Part model, mm, in its own coordinate system. A direction names the side the tool comes from. Coordinates: 2 decimals unless noted, no trailing zeros. Order: outer loops, then holes, each group sorted by start corner. A loop starts at its lowest first (then second) coordinate and runs counter-clockwise, first axis right, second up. Notation, with made-up numbers: (-5, 53) - (3, 53) arc R23 cw to (3, 77) - close; hole circle Ø11 at (-13.75, -22.5). An arc over 180 degrees is marked (long way). Use a Markdown table: item, result. Add a question column.
1) Saw through at B-B on z = -1. List the corners of the cut face in (x, y) (1 decimal).
2) Wall check: L1, parallel to X at y = 35.5, z = -5.5; L2, parallel to X at y = -8.5, z = -4.5; L3, parallel to Y at x = -57.5, z = -6. Give the ranges that are in metal, low to high. Write a range as [from, to].
3) Tool access for faces 1 (the face through (48.09, 6.6, -4.42)), 2 (the face through (76.2, -1, -3)), 3 (the face through (40.66, 4.95, -1.29)): list every direction of +Z, -Z, +X, -X, +Y, -Y with a clear straight run to the whole face (end or side of a thin tool).
4) Two-plate mould, pull along X, no slides. Class faces 4 (the face through (-65.206, -9.31, -2.417)), 5 (the face through (-76.2, -1, -3)), 6 (the face through (-38.44, 38.14, -4.42)), 7 (the face through (-1, -50.8, -3)): +X half, -X half, draft (parallel to the pull), parting line (faces both ways), or undercut.
5) Saw through at C-C on x = -9.5. Count the separate pieces of the cut face and the enclosed holes in it, then the cut area to 3 significant figures.
6) Saw through at A-A on y = -0.5. List the corners of the cut face in (x, z).
```python
from build123d import *

# Parameters (mm, degrees)
F0_W     = 152.4
F0_H     = 101.6
F0_R     = 4.7625
F2_DEPTH = 6.35
F3_DEPTH = 25.4
F4_SIZE  = 2.54


with BuildPart() as f2:
    # F0 (on Top) → F2 (new body)
    with BuildSketch(Plane.XY):
        Rectangle(F0_W, F0_H)
        with Locations((-60.325, -9.525)):
            Circle(F0_R, mode=Mode.SUBTRACT)
        with Locations((-34.925, -9.525)):
            Circle(F0_R, mode=Mode.SUBTRACT)
        with Locations((-9.525, -9.525)):
            Circle(F0_R, mode=Mode.SUBTRACT)
        with Locations((-60.325, 34.925)):
            Circle(F0_R, mode=Mode.SUBTRACT)
        with Locations((-34.925, 34.925)):
            Circle(F0_R, mode=Mode.SUBTRACT)
        with Locations((-9.525, 34.925)):
            Circle(F0_R, mode=Mode.SUBTRACT)
    extrude(amount=-F2_DEPTH)

    # F1 (on face) → F3 (cut)
    with BuildSketch(Plane.XY):
        with BuildLine():
            Line((51.546737, -5.978524), (44.529635, 19.542772))
            ThreePointArc((44.529635, 19.542772), (40.626513, 21.762431), (38.406854, 17.859308))
            Line((38.406854, 17.859308), (45.423956, -7.661988))
            ThreePointArc((45.423956, -7.661988), (49.327078, -9.881647), (51.546737, -5.978524))
        make_face()
    extrude(amount=-F3_DEPTH, mode=Mode.SUBTRACT)

    # F4
    f4_edges = [f2.edges().sort_by_distance(p)[0] for p in [
        (-65.0875, 34.925, 0),
        (-39.6875, 34.925, 0),
        (-14.2875, 34.925, 0),
        (-14.2875, -9.525, 0),
        (-39.6875, -9.525, 0),
        (-65.0875, -9.525, 0),
        (41.915405, 5.09866, 0),
    ]]
    chamfer(f4_edges, length=F4_SIZE)


solid = f2.part
```
Results are:
| question | item | result |
|---|---|---|
| 1 | outline | (-76.2, -50.8) - (76.2, -50.8) - (76.2, 50.8) - (-76.2, 50.8) - close; hole circle Ø12.6 at (-60.3, -9.5); hole circle Ø12.6 at (-60.3, 34.9); hole circle Ø12.6 at (-34.9, -9.5); hole circle Ø12.6 at (-34.9, 34.9); hole circle Ø12.6 at (-9.5, -9.5); hole circle Ø12.6 at (-9.5, 34.9); hole (36.9, 17.5) - (43.9, -8.1) arc R4.7 ccw to (53, -5.6) - (46, 20) arc R4.7 ccw to start |
| 2 | L1 | [-76.2, -65.05], [-55.6, -39.65], [-30.2, -14.25], [-4.8, 76.2] |
| 2 | L2 | [-76.2, -64.98], [-55.67, -39.58], [-30.27, -14.18], [-4.87, 45.79], [51.18, 76.2] |
| 2 | L3 | [-50.8, -13.36], [-5.69, 31.09], [38.76, 50.8] |
| 3 | face 1 | +Z, -Z |
| 3 | face 2 | +Z, -Z, +X, +Y, -Y |
| 3 | face 3 | +Z |
| 4 | face 4 | undercut |
| 4 | face 5 | -X half |
| 4 | face 6 | undercut |
| 4 | face 7 | draft |
| 5 | separate pieces | 3 |
| 5 | enclosed holes | 0 |
| 5 | area | 511 mm2 |
| 6 | outline | (-76.2, -6.35) - (43.45, -6.35) - (43.45, -2.54) - (40.82, 0) - (-76.2, 0) - close; (50.04, -6.35) - (76.2, -6.35) - (76.2, 0) - (52.67, 0) - (50.04, -2.54) - close |
